from build123d import *
from build123d.topology import SkipClean

# Parameters (mm, degrees)
SKETCH_1_R      = 12.5
EXTRUDE_1_DEPTH = 2
EXTRUDE_2_DEPTH = 2
EXTRUDE_3_DEPTH = 2
SKETCH_5_R      = 2.5
SKETCH_5_R_2    = 1.5
EXTRUDE_4_DEPTH = 2
EXTRUDE_START   = 2
SKETCH_6_R      = 1.5
SKETCH_6_R_2    = 1
SKETCH_6_R_3    = 2.5
EXTRUDE_5_DEPTH = 2


with BuildPart() as part:
    # Эскиз1 → Бобышка-Вытянуть1 (new body)
    with BuildSketch(Plane(origin=(0, 0, 0), x_dir=(1, 0, 0), z_dir=(0, 1, 0))):
        with Locations(Location((0, 0, 0), (0, 0, 270))):
            Circle(SKETCH_1_R)
    extrude(amount=EXTRUDE_1_DEPTH)

    # Эскиз2 → Бобышка-Вытянуть2 (add)
    with BuildSketch(Plane(origin=(0, 2, 0), x_dir=(1, 0, 0), z_dir=(0, 1, 0))):
        with BuildLine():
            ThreePointArc((-11.328847338, 5.282728272), (-12.203700089, 2.705495174), (-12.5, 0))
            Line((-12.5, 0), (-10.5, 0))
            ThreePointArc((-10.5, 0), (-10.251108075, 2.272615946), (-9.516231764, 4.437491748))
            Line((-9.516231764, 4.437491748), (-11.328847338, 5.282728272))
        make_face()
        with BuildLine():
            ThreePointArc((-12.5, 0), (-12.203700089, -2.705495174), (-11.328847338, -5.282728272))
            Line((-11.328847338, -5.282728272), (-9.516231764, -4.437491748))
            ThreePointArc((-9.516231764, -4.437491748), (-10.251108075, -2.272615946), (-10.5, 0))
            Line((-10.5, 0), (-12.5, 0))
        make_face()
        with BuildLine():
            Line((6.782329983, -10.5), (0, -10.5))
            ThreePointArc((0, -10.5), (-1.370525018, -10.410171044), (-2.717599974, -10.142221176))
            Line((-2.717599974, -10.142221176), (-3.235238064, -12.074072829))
            ThreePointArc((-3.235238064, -12.074072829), (1.940332855, -12.348486078), (6.782329983, -10.5))
        make_face()
        with BuildLine():
            Line((0, 10.5), (6.782329983, 10.5))
            ThreePointArc((6.782329983, 10.5), (1.940332855, 12.348486078), (-3.235238064, 12.074072829))
            Line((-3.235238064, 12.074072829), (-2.717599974, 10.142221176))
            ThreePointArc((-2.717599974, 10.142221176), (-1.370525018, 10.410171044), (0, 10.5))
        make_face()
    extrude(amount=EXTRUDE_2_DEPTH)

    # Эскиз4 → Бобышка-Вытянуть3 (add)
    with BuildSketch(Plane(origin=(0, 4, 0), x_dir=(1, 0, 0), z_dir=(0, 1, 0))):
        with BuildLine():
            ThreePointArc((-11.328847338, -5.282728272), (-3.460156945, -12.011549189), (6.782329983, -10.5))
            Line((6.782329983, -10.5), (-2.598361206, -7.035518392))
            ThreePointArc((-2.598361206, -7.035518392), (-7.5, 0), (-2.598361206, 7.035518392))
            Line((-2.598361206, 7.035518392), (6.782329983, 10.5))
            ThreePointArc((6.782329983, 10.5), (-3.460156945, 12.011549189), (-11.328847338, 5.282728272))
            Line((-11.328847338, 5.282728272), (-9.516231764, 4.437491748))
            ThreePointArc((-9.516231764, 4.437491748), (-10.5, 0), (-9.516231764, -4.437491748))
            Line((-9.516231764, -4.437491748), (-11.328847338, -5.282728272))
        make_face()
        with BuildLine():
            Line((-9.516231764, 4.437491748), (-11.328847338, 5.282728272))
            ThreePointArc((-11.328847338, 5.282728272), (-12.5, 0), (-11.328847338, -5.282728272))
            Line((-11.328847338, -5.282728272), (-9.516231764, -4.437491748))
            ThreePointArc((-9.516231764, -4.437491748), (-10.5, 0), (-9.516231764, 4.437491748))
        make_face()
    extrude(amount=EXTRUDE_3_DEPTH)

    # Эскиз5 → Бобышка-Вытянуть4 (add)
    with BuildSketch(Plane.XZ):
        with BuildLine():
            Line((-20.2, 10.25), (-20.2, -10.25))
            ThreePointArc((-20.2, -10.25), (-17.284002551, -15.935149353), (-10.965450526, -16.883761274))
            Line((-10.965450526, -16.883761274), (3.990266919, -11.846002276))
            ThreePointArc((3.990266919, -11.846002276), (12.5, 0), (3.990266919, 11.846002276))
            Line((3.990266919, 11.846002276), (-10.965450526, 16.883761274))
            ThreePointArc((-10.965450526, 16.883761274), (-17.284002551, 15.935149353), (-20.2, 10.25))
        make_face()
        with Locations(Location((-13.2, 10.25, 0), (0, 0, 270))):
            Circle(SKETCH_5_R, mode=Mode.SUBTRACT)
        with Locations(Location((-13.2, -10.25, 0), (0, 0, 270))):
            Circle(SKETCH_5_R_2, mode=Mode.SUBTRACT)
    extrude(amount=-EXTRUDE_4_DEPTH)

    # Эскиз6 → Бобышка-Вытянуть5 (add)
    with SkipClean():  # the faces are left unmerged after this step: merging them gives an invalid solid
        with BuildSketch(Plane.XZ.offset(EXTRUDE_START)):
            with BuildLine():
                Line((3.990266919, 11.846002276), (-10.965450526, 16.883761274))
                ThreePointArc((-10.965450526, 16.883761274), (-17.284002551, 15.935149353), (-20.2, 10.25))
                Line((-20.2, 10.25), (-20.2, -10.25))
                ThreePointArc((-20.2, -10.25), (-17.284002551, -15.935149353), (-10.965450526, -16.883761274))
                Line((-10.965450526, -16.883761274), (3.990266919, -11.846002276))
                ThreePointArc((3.990266919, -11.846002276), (12.5, 0), (3.990266919, 11.846002276))
            make_face()
            with Locations(Location((-13.2, -10.25, 0), (0, 0, 270))):
                Circle(SKETCH_6_R, mode=Mode.SUBTRACT)
            with Locations(Location((-8.2, 10.25, 0), (0, 0, 270))):
                Circle(SKETCH_6_R_2, mode=Mode.SUBTRACT)
            with Locations(Location((-13.2, 5.25, 0), (0, 0, 270))):
                Circle(SKETCH_6_R_2, mode=Mode.SUBTRACT)
            with Locations(Location((-18.2, 10.25, 0), (0, 0, 270))):
                Circle(SKETCH_6_R_2, mode=Mode.SUBTRACT)
            with Locations(Location((-13.2, 15.25, 0), (0, 0, 270))):
                Circle(SKETCH_6_R_2, mode=Mode.SUBTRACT)
            with Locations(Location((-13.2, 10.25, 0), (0, 0, 270))):
                Circle(SKETCH_6_R_3, mode=Mode.SUBTRACT)
        extrude(amount=-EXTRUDE_5_DEPTH)


solid = part.part
Geometry check sheet. Reference: the model listing, model coordinates, mm. A direction names the side the tool comes from. Give positions to 0.01 mm unless a question says otherwise; leave off trailing zeros. Loops run counter-clockwise (first coordinate to the right, second up) from the corner with the lowest first, then second, coordinate; pieces in that order, holes last. Notation, with made-up numbers: M 65,27 L 98,27 A20 cw 98,40 Z; hole C -13.75,47.25 d10. An arc over 180 degrees is marked long. Write each question's results on one line, items separated by ' | '.
1) Section check C-C, the plane z = -6.5. Record the boundary of the cut face in (x, y), plus the area to 3 significant figures.
Answers follow:
outline: M -20.2,-2 L 10.68,-2 L 10.68,2 L -20.2,2 Z; M -10.68,4 L -3.74,4 L -3.74,6 L -10.68,6 Z | area: 137 mm2
2) Thickness scan on line 1 (Y direction, x = -6, z = -8.5); line 2 (Y direction, x = -10.5, z = 13); line 3 (X direction, y = 0.7, z = 10.25). Record the ranges inside material, lowest first.
Answers follow:
line 1: -2 to 2, 4 to 6 | line 2: -2 to 2 | line 3: -20.2 to -15.7, -10.7 to 7.15
3) Section check A-A, the plane y = 3.5. Record the boundary of the cut face in (x, z), plus the area to 3 significant figures.
Answers follow:
outline: M -11.33,-5.28 L -9.52,-4.44 A10.5 cw -9.52,4.44 L -11.33,5.28 A12.5 ccw Z; M -3.24,-12.07 A12.5 ccw 6.78,-10.5 L 0,-10.5 A10.5 cw -2.72,-10.14 Z; M -3.24,12.07 L -2.72,10.14 A10.5 cw 0,10.5 L 6.78,10.5 A12.5 ccw Z | area: 50.5 mm2
4) Release check for a two-part mould opening along Y. For faces 1 (the face through (-1.351, 2.986, 10.413)), 2 (the face through (-8.81, -1.01, 11.04)), 3 (the face through (-4, -2, 0)) record: +Y half, -Y half, draft (parallel to the pull), parting line (faces both ways), or undercut.
Answers follow:
face 1: undercut | face 2: draft | face 3: -Y half
5) Tool access check on faces 4 (the face through (-10.44, 2.99, 4.87)), 5 (the face through (3, 3, 10.5)), 6 (the face through (2.026, 4.986, -8.744)), 7 (the face through (-2.98, 2.99, -11.12)). Record the directions out of +Z, -Z, +X, -X, +Y, -Y that give a thin tool (end or side, any length) a straight path to the whole face; none if there is none.
Answers follow:
face 4: +Z, +X | face 5: +X | face 6: +X, +Y | face 7: -X
6) Section check B-B, the plane y = -0.5. Record the boundary of the cut face in (x, z), plus the area to 3 significant figures.
Answers follow:
outline: M -20.2,-10.25 A7 ccw -10.97,-16.88 L 3.99,-11.85 A12.5 ccw 3.99,11.85 L -10.97,16.88 A7 ccw -20.2,10.25 Z; hole C -18.2,10.25 d2; hole C -13.2,10.25 d5; hole C -13.2,-10.25 d3; hole C -13.2,5.25 d2; hole C -13.2,15.25 d2; hole C -8.2,10.25 d2 | area: 835 mm2
7) Gauge pin test, flat ends, axial feed: pin 1 (2.5 mm diameter, centred on x = -13.2, z = 15.25, fed in from -Y); pin 2 (0.6 mm diameter, centred on x = -13.5, z = 15.5, fed in from -Y); pin 3 (1.5 mm diameter, centred on x = 5, y = 2, fed in from -Z); pin 4 (2 mm diameter, centred on x = 3, y = 3, fed in from +Z). Record the tip position at first contact, or that the pin passes through.
Answers follow:
pin 1: y = -2 | pin 2: y = 0 | pin 3: z = -11.76 | pin 4: z = 12.34
8) Section check D-D, the plane x = -8.2. Record the boundary of the cut face in (y, z), plus the area to 3 significant figures.
Answers follow:
outline: M -2,-15.95 L 2,-15.95 L 2,15.95 L -2,15.95 L -2,11.25 L 0,11.25 L 0,9.25 L -2,9.25 Z; M 4,-9.43 L 6,-9.43 L 6,9.43 L 4,9.43 Z | area: 161 mm2
